Here's how the part is built. I have some questions about the finished solid (model axes, mm). Face numbers are marked on the shaded views. Give positions to 0.01 mm unless a question says otherwise; leave off trailing zeros. Order: outer loops, then holes, each group sorted by start corner. A loop starts at its lowest first (then second) coordinate and runs counter-clockwise, first axis right, second up.
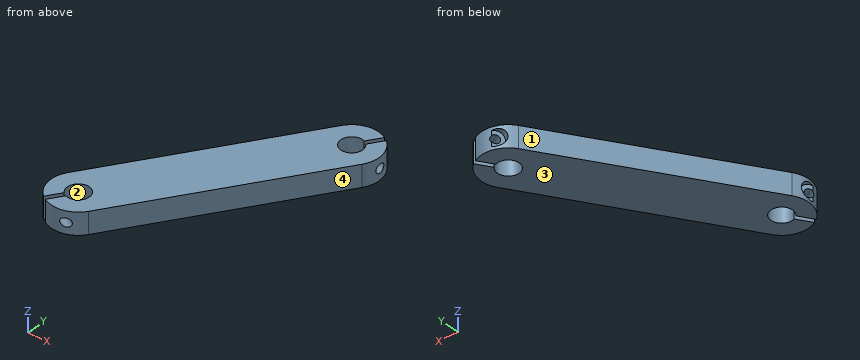
from build123d import *

# Parameters (mm, degrees)
SKETCH1_R                 = 3.175
BOSS_EXTRUDE1_DEPTH       = 6.35
CUT_EXTRUDE1_DEPTH        = 210.56202617
CBORE_FOR_2_1_D           = 2.4384
CBORE_FOR_2_1_CBORE_D     = 4.7625
CBORE_FOR_2_1_CBORE_DEPTH = 2.3114


with BuildPart() as part:
    # Sketch1 → Boss-Extrude1 (new body)
    with BuildSketch(Plane.XY):
        with BuildLine():
            Line((47.587554204, 128.214676374), (82.223145852, 182.092263381))
            ThreePointArc((82.223145852, 182.092263381), (93.192263381, 184.476854148), (95.576854148, 173.507736619))
            Line((95.576854148, 173.507736619), (60.941262501, 119.630149611))
            ThreePointArc((60.941262501, 119.630149611), (49.972144971, 117.245558844), (47.587554204, 128.214676374))
        make_face()
        with Locations((88.9, 177.8)):
            Circle(SKETCH1_R, mode=Mode.SUBTRACT)
        with Locations((54.264408352, 123.922412992)):
            Circle(SKETCH1_R, mode=Mode.SUBTRACT)
    extrude(amount=BOSS_EXTRUDE1_DEPTH)

    # Sketch2 → Cut-Extrude1 (cut, through all)
    with BuildSketch(Plane.XY.offset(6.35)):
        with BuildLine():
            Line((92.644357759, 184.79883499), (90.048068488, 180.760162791))
            ThreePointArc((90.048068488, 180.760162791), (90.616905352, 180.470741659), (91.116365152, 180.07340065))
            Line((91.116365152, 180.07340065), (93.712654423, 184.112072849))
            ThreePointArc((93.712654423, 184.112072849), (93.192263381, 184.476854148), (92.644357759, 184.79883499))
        make_face()
        with BuildLine():
            Line((52.0480432, 121.649012343), (49.451753929, 117.610340143))
            ThreePointArc((49.451753929, 117.610340143), (49.972144971, 117.245558844), (50.520050593, 116.923578002))
            Line((50.520050593, 116.923578002), (53.116339864, 120.962250202))
            ThreePointArc((53.116339864, 120.962250202), (52.547503, 121.251671333), (52.0480432, 121.649012343))
        make_face()
    extrude(amount=-CUT_EXTRUDE1_DEPTH, mode=Mode.SUBTRACT)

    # CBORE for #2 _1 (through all)
    with Locations(Plane(origin=(-24.649417325, 15.846053995, 0), x_dir=(0, 0, 1), z_dir=(-0.8411784753765535, 0.540757591313499, 0))):
        with Locations((3.175, 202.371942019), (3.175, 128.847697951)):
            CounterBoreHole(CBORE_FOR_2_1_D / 2, CBORE_FOR_2_1_CBORE_D / 2, CBORE_FOR_2_1_CBORE_DEPTH)


solid = part.part
Q1. If we section it at A-A on x = 88.9: Give the number of separate pieces and of enclosed holes in the cut face, plus the area to 3 significant figures.
Filled sheet:
separate pieces: 2
enclosed holes: 1
area: 97.7 mm2
Q2. If we section it at C-C on y = 141.5: List the corners of the cut face in (x, z) for me, plus the area to 3 significant figures.
Filled sheet:
outline: (56.13, 0) - (75, 0) - (75, 6.35) - (56.13, 6.35) - close
area: 120 mm2
Q3. I'm going to push flat-ended pins straight in: P1, Ø5.5, axis at x = 54.26, y = 123.92, coming from the -Z side; P2, Ø3, axis at x = 52.5, z = 3.5, coming from the -Y side. Where does each tip first touch, or does it pass through?
Filled sheet:
P1: passes through
P2: stops at y = 115.99
Q4. If we section it at D-D on x = 65.5: List the corners of the cut face in (y, z) for me, plus the area to 3 significant figures.
Filled sheet:
outline: (126.72, 0) - (156.08, 0) - (156.08, 6.35) - (126.72, 6.35) - close
area: 186 mm2
Q5. I need wall thicknesses on L1, parallel to Y at x = 88.9, z = 4.25 (1 decimal); L2, parallel to Y at x = 88.9, z = 3.5 (1 decimal); L3, parallel to X at y = 121.5, z = 2.25. Which ranges of each line are inside material? Lowest first, please.
Filled sheet:
L1: y = 163.1 to 174.6, 181 to 182.7, 184.1 to 185.7
L2: y = 163.1 to 174.6, 181 to 182, 184.8 to 185.7
L3: x = 46.71 to 47.8, 50.74 to 51.95, 56.32 to 62.14
Q6. Thinking about a two-plate mould opening in X: for the marked faces 1, 2, 3 and 4, which applies, released by +X, released by -X, zero draft, split by the parting line, or undercut?
Filled sheet:
face 1: released by -X
face 2: undercut
face 3: zero draft
face 4: released by +X
